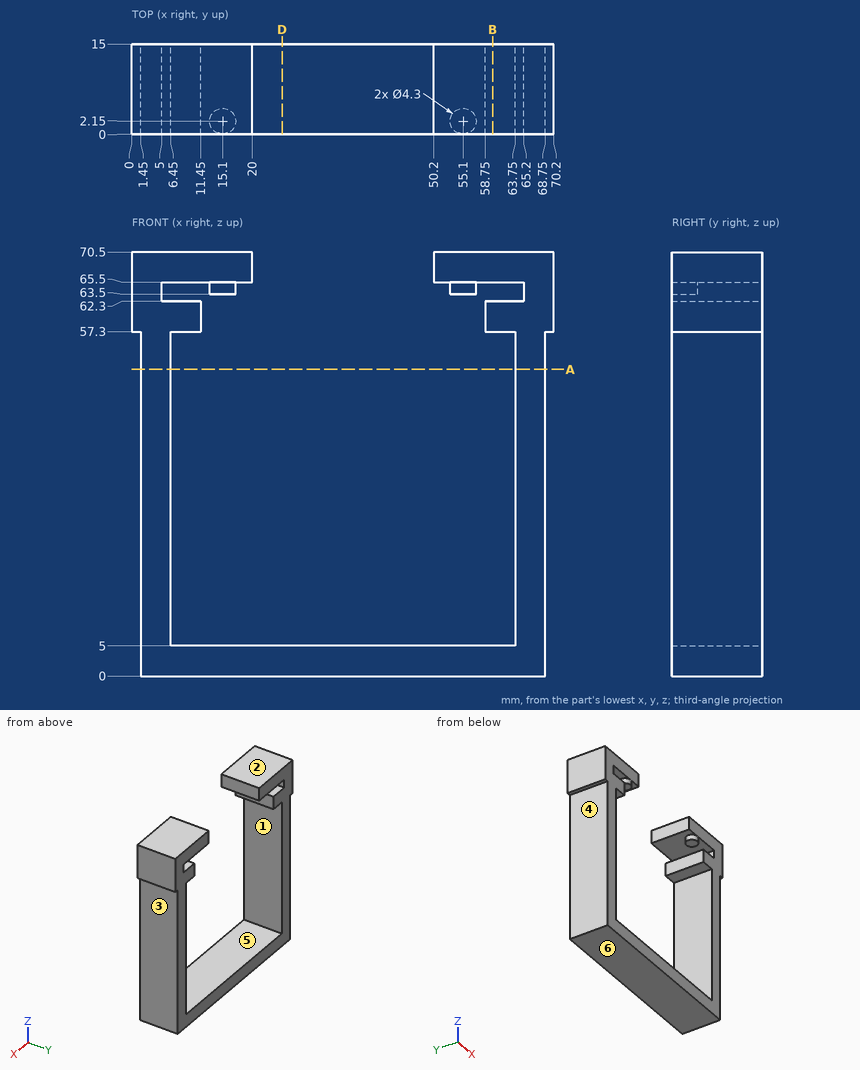
Study the drawing (mm; zero at the part's minimum x, y, z) and answer. A direction names the side the tool comes from. Give positions to 0.01 mm unless a question says otherwise; leave off trailing zeros. Order: outer loops, then holes, each group sorted by start corner. A loop starts at its lowest first (then second) coordinate and runs counter-clockwise, first axis right, second up. Notation, with made-up numbers: (71, 29) - (123, 29) arc R21 ccw to (123, 56) - close; hole circle Ø2 at (-32, 4). An arc over 180 degrees is marked (long way). Use one line per item in the form item = value. Start each with the question number.
(1) Flat-ended cylindrical pins translate along their axes: pin 1 Ø2 at (x, y) = (40.5, 7.5) entering from +Z; pin 2 Ø4.5 at (y, z) = (8, 38) entering from +X; pin 3 Ø4.5 at (x, y) = (15, 2.5) entering from -Z; pin 4 Ø1 at (x, z) = (7.5, 17) entering from +Y. Find the tip coordinate at first contact, or state that the pin passes through.
(2) A cutting plane is placed at A-A, the plane z = 51. Write down the section's boundary in (x, y).
(3) For the marked faces 1, 2 and 3, determine the directions among +Z, -Z, +X, -X, +Y, -Y from which every point of the face is accessible in a straight line to the end or side of a thin tool.
(4) Consider line 1 (Z direction, x = 9.5, y = 12.75); line 2 (X direction, y = 12, z = 43); line 3 (Z direction, x = 11.5, y = 11.75). Determine where each line is inside the solid, lowest interval first. Write a range as from..to.
(5) A cutting plane is placed at B-B, the plane x = 60. Write down the section's boundary in (y, z), then the cut area to 3 significant figures.
(6) A cutting plane is placed at D-D, the plane x = 25. Write down the section's boundary in (y, z), then the cut area to 3 significant figures.
(7) The mould has two halves that part along X. Classify the marked faces 4, 5 and 6: released by +X, released by -X, zero draft, split by the parting line, or undercut.
Ans:
q1.pin_1 = 5
q1.pin_2 = 68.75
q1.pin_3 = 0
q1.pin_4 = through
q2.outline = (1.45, 0) - (6.45, 0) - (6.45, 15) - (1.45, 15) - close; (63.75, 0) - (68.75, 0) - (68.75, 15) - (63.75, 15) - close
q3.face_1 = +Y, -Y
q3.face_2 = +Z, +X, -X, +Y, -Y
q3.face_3 = -Z, +X, +Y, -Y
q4.line_1 = 0..5, 57.3..62.3, 65.5..70.5
q4.line_2 = 1.45..6.45, 63.75..68.75
q4.line_3 = 0..5, 65.5..70.5
q5.outline = (0, 0) - (15, 0) - (15, 5) - (0, 5) - close; (0, 57.3) - (15, 57.3) - (15, 62.3) - (0, 62.3) - close; (0, 65.5) - (15, 65.5) - (15, 70.5) - (0, 70.5) - close
q5.area = 225 mm^2
q6.outline = (0, 0) - (15, 0) - (15, 5) - (0, 5) - close
q6.area = 75.0 mm^2
q7.face_4 = released by -X
q7.face_5 = undercut
q7.face_6 = zero draft
